```python
from build123d import *

# Parameters (mm, degrees)
SKETCH1_W           = 40
SKETCH1_H           = 100
SKETCH1_H_2         = 60
BOSS_EXTRUDE1_DEPTH = 2
SKETCH2_R           = 3
CUT_EXTRUDE1_DEPTH  = 5
CHAMFER1_SIZE       = 3


with BuildPart() as part:
    # Sketch1 → Boss-Extrude1 (new body, symmetric)
    with BuildSketch(Plane.XY):
        Rectangle(SKETCH1_W, SKETCH1_H)
        Polygon((60, 30), (20, 50), (20, 30), align=None)
        with Locations((40, 0)):
            Rectangle(SKETCH1_W, SKETCH1_H_2)
        Polygon((20, -50), (60, -30), (20, -30), align=None)
    extrude(amount=BOSS_EXTRUDE1_DEPTH, both=True)

    # Sketch2 → Cut-Extrude1 (cut, through all)
    with BuildSketch(Plane.XY.offset(2)):
        with Locations((-10, 20)):
            Circle(SKETCH2_R)
        with Locations((-10, -20)):
            Circle(SKETCH2_R)
        with Locations((10, -40)):
            Circle(SKETCH2_R)
        with Locations((40, -20)):
            Circle(SKETCH2_R)
        with Locations((30, 20)):
            Circle(SKETCH2_R)
        with Locations((50, 20)):
            Circle(SKETCH2_R)
        with Locations((10, 40)):
            Circle(SKETCH2_R)
    extrude(amount=-CUT_EXTRUDE1_DEPTH, mode=Mode.SUBTRACT)

    # Chamfer1
    chamfer1_edges = [part.edges().sort_by_distance(p)[0] for p in [
        (37, -20, 2),
        (7, -40, 2),
        (-13, -20, 2),
        (7, 40, 2),
        (27, 20, 2),
        (47, 20, 2),
        (-13, 20, 2),
    ]]
    chamfer(chamfer1_edges, length=CHAMFER1_SIZE)


solid = part.part
```
Geometry check sheet. Reference: the model listing, model coordinates, mm. Coordinates: 2 decimals unless noted, no trailing zeros. Loops run counter-clockwise (first coordinate to the right, second up) from the corner with the lowest first, then second, coordinate; pieces in that order, holes last.
Item 1: Sectioned sample at D-D, the plane x = 10. Record the boundary of the cut face in (y, z), then the cut area to 3 significant figures.
Item 2: Release check for a two-part mould opening along X. For faces 1 (the face through (40, 40, 0)), 2 (the face through (0, -50, 0)), 3 (the face through (27, 20.1, -1.5)), 4 (the face through (53, 20.945, -0.854)) record: released by +X, released by -X, zero draft, split by the parting line, or undercut.
Item 3: Thickness scan on line 1 (Y direction, x = 10, z = -1.5); line 2 (Y direction, x = -10, z = -1.7); line 3 (Y direction, x = 38, z = -1.3). Record the ranges inside material, lowest first.
Item 4: Sectioned sample at C-C, the plane y = -20. Record the boundary of the cut face in (x, z).
Item 5: Go/stop test with flat-tipped pins: pin 1 Ø5.5 at (x, y) = (-10, -20) entering from -Z (3 decimals); pin 2 Ø2 at (x, z) = (23, -1) entering from -Y; pin 3 Ø9.5 at (x, y) = (10, 40) entering from +Z; pin 4 Ø7 at (x, y) = (40, -20) entering from +Z. Record where each tip stops, or that it passes through.
Item 6: Sectioned sample at B-B, the plane x = 40. Record the boundary of the cut face in (y, z), then the cut area to 3 significant figures.
Item 7: Sectioned sample at A-A, the plane y = 40. Record the boundary of the cut face in (x, z), then the cut area to 3 significant figures.
Check result:
1. outline: (-50, -2) - (-43, -2) - (-43, -1) - (-46, 2) - (-50, 2) - close; (-37, -2) - (37, -2) - (37, -1) - (34, 2) - (-34, 2) - (-37, -1) - close; (43, -2) - (50, -2) - (50, 2) - (46, 2) - (43, -1) - close
1. area: 334 mm2
2. face 1: released by +X
2. face 2: zero draft
2. face 3: undercut
2. face 4: undercut
3. line 1: y = -50 to -43, -37 to 37, 43 to 50
3. line 2: y = -50 to -23, -17 to 17, 23 to 50
3. line 3: y = -41 to -22.24, -17.76 to 41
4. outline: (-20, -2) - (-13, -2) - (-13, -1) - (-16, 2) - (-20, 2) - close; (-7, -2) - (37, -2) - (37, -1) - (34, 2) - (-4, 2) - (-7, -1) - close; (43, -2) - (60, -2) - (60, 2) - (46, 2) - (43, -1) - close
5. pin 1: passes through
5. pin 2: stops at y = -49
5. pin 3: stops at z = 0.75
5. pin 4: stops at z = -0.5
6. outline: (-40, -2) - (-23, -2) - (-23, -1) - (-26, 2) - (-40, 2) - close; (-17, -2) - (40, -2) - (40, 2) - (-14, 2) - (-17, -1) - close
6. area: 287 mm2
7. outline: (-20, -2) - (7, -2) - (7, -1) - (4, 2) - (-20, 2) - close; (13, -2) - (40, -2) - (40, 2) - (16, 2) - (13, -1) - close
7. area: 207 mm2
